The drawing under review shows one solid part. Ordinate dimensions are in mm from its lowest x, y, z. A direction names the side the tool comes from. Coordinates: 2 decimals unless noted, no trailing zeros. Loops run counter-clockwise (first coordinate to the right, second up) from the corner with the lowest first, then second, coordinate; pieces in that order, holes last. Notation, with made-up numbers: M 58.25,-15.75 L 84.25,-15.75 A11 ccw 84.25,-9.75 Z; hole C 61.5,8 d10. An arc over 180 degrees is marked long. Put each result on its own line as item: value.
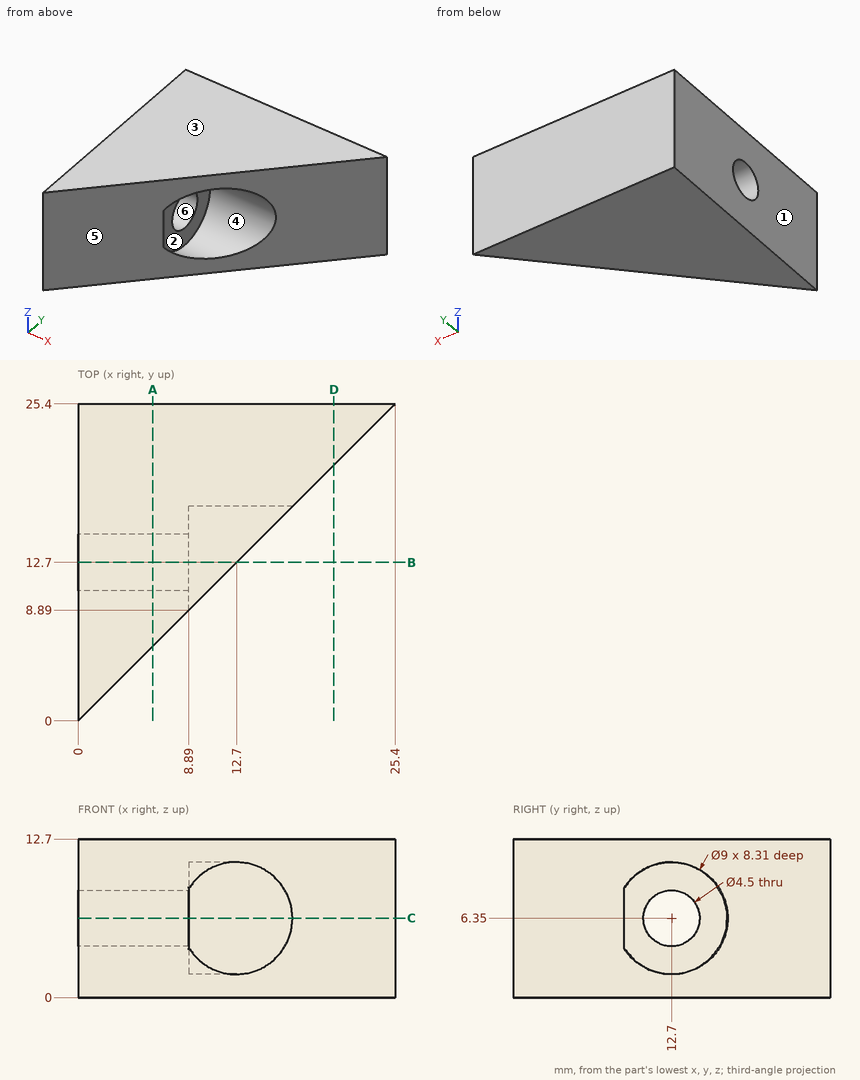
(1) Add section B-B (y = 12.7). Write out the cut boundary in (x, z), plus the area to 3 significant figures.
Determined:
outline: M 0,0 L 12.7,0 L 12.7,1.85 L 8.89,1.85 L 8.89,4.1 L 0,4.1 Z; M 0,8.6 L 8.89,8.6 L 8.89,10.85 L 12.7,10.85 L 12.7,12.7 L 0,12.7 Z
area: 87.0 mm^2
(2) Add section C-C (z = 6.35). Write out the cut boundary in (x, y), plus the area to 3 significant figures.
Determined:
outline: M 0,0 L 8.89,8.89 L 8.89,10.45 L 0,10.45 Z; M 0,14.95 L 8.89,14.95 L 8.89,17.2 L 17.2,17.2 L 25.4,25.4 L 0,25.4 Z
area: 248 mm^2
(3) Draft analysis for pull direction Z (two halves, no side actions). For the marked faces 3, 4, 5 and 6, state which applies: +Z half, -Z half, draft (parallel to the pull), parting line (faces both ways), or undercut.
Determined:
face 3: +Z half
face 4: undercut
face 5: draft
face 6: undercut
(4) Tool access review of the marked faces 1 and 2: name each direction out of +Z, -Z, +X, -X, +Y, -Y from which nothing blocks a thin tool from reaching the whole face with its end or side.
Determined:
face 1: +Z, -Z, -X, +Y, -Y
face 2: +X
(5) For pin 1 (2.5 mm diameter, centred on y = 14, z = 6, fed in from +X); pin 2 (5 mm diameter, centred on x = 12, z = 11, fed in from -Y), all flat-tipped, find the tip position at first contact; note any pin that passes through.
Determined:
pin 1: stops at x = 8.89
pin 2: stops at y = 9.5
(6) Wall thickness on line 1 along Y through (x, z) = (14.25, 6.35); line 2 along X through (y, z) = (15.5, 3); line 3 along Y through (x, z) = (3, 6.35): over which ranges is each line inside the solid? List them lowest first. Write a range as [from, to].
Determined:
line 1: y = [17.2, 25.4]
line 2: x = [0, 8.89]
line 3: y = [3, 10.45], [14.95, 25.4]
(7) Add section D-D (x = 20.5). Write out the cut boundary in (y, z).
Determined:
outline: M 20.5,0 L 25.4,0 L 25.4,12.7 L 20.5,12.7 Z
(8) Add section A-A (x = 6). Write out the cut boundary in (y, z), plus the area to 3 significant figures.
Determined:
outline: M 6,0 L 25.4,0 L 25.4,12.7 L 6,12.7 Z; hole C 12.7,6.35 d4.5
area: 230 mm^2
